from build123d import *

# Parameters (mm, degrees)
ESQUISSE1_R        = 10.75
BOSS_EXTRU_1_DEPTH = 6
ESQUISSE3_R        = 0.7
BOSS_EXTRU_2_DEPTH = 3
CONG_1_R           = 1


with BuildPart() as part:
    # Esquisse1 → Boss.-Extru.1 (new body)
    with BuildSketch(Plane.XY):
        Circle(ESQUISSE1_R)
    extrude(amount=BOSS_EXTRU_1_DEPTH)

    # Esquisse3 → Boss.-Extru.2 (add)
    with BuildSketch(Plane(origin=(0, 0, 0), x_dir=(-1, 0, 0), z_dir=(0, 0, -1))):
        with Locations(Location((-2.5, 0, 0), (0, 0, 180))):
            Circle(ESQUISSE3_R)
        with Locations(Location((2.5, 0, 0), (0, 0, 180))):
            Circle(ESQUISSE3_R)
    extrude(amount=BOSS_EXTRU_2_DEPTH)

    # Congé1
    cong_1_edges = [part.edges().sort_by_distance(p)[0] for p in [
        (-10.75, 0, 0),
        (-10.75, 0, 6),
    ]]
    fillet(cong_1_edges, radius=CONG_1_R)


solid = part.part
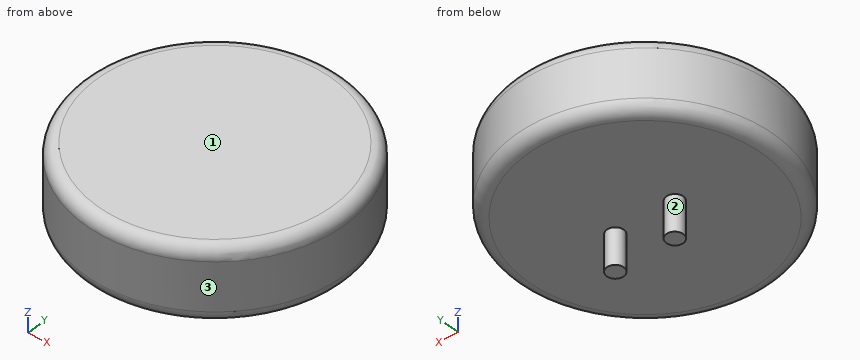
Can you work these out from the model? Positions are in its coordinate system, mm. Face numbers are marked on the shaded views. Round coordinates to 2 decimals unless told otherwise and drop trailing zeros. Write each loop counter-clockwise with the first axis right and the second up, starting at its lowest first coordinate (ties: lowest second). Pieces come first, ordered by that corner, then holes. Notation, with made-up numbers: (-24, 74.5) - (35, 74.5) arc R23 cw to (35, 92.5) - close; hole circle Ø4 at (-27, -8.75). An arc over 180 degrees is marked (long way). Write each question's results on one line, items separated by ' | '. Start each with the question number.
1) Please list where these lines run through material, in increasing order: line 1 (Z direction, x = 4.5, y = -4); line 2 (Y direction, x = -4.75, z = 0.5); line 3 (Y direction, x = 9.5, z = 1.5).
2) Suppose I cut it at C-C (z = -0.5). List the corners of the cut face in (x, y) for me, and give its area (3 significant figures).
3) Suppose I cut it at D-D (z = 2.25). List the corners of the cut face in (x, y) for me, and give its area (3 significant figures).
4) We'd pull the mould along X, two halves only. Please class the marked faces 1, 2 and 3: released by +X, released by -X, zero draft, split by the parting line, or undercut.
5) For pin 1 Ø2 at (x, z) = (3, 1) entering from -Y; pin 2 Ø1.5 at (x, z) = (1, 3) entering from -Y, each with a flat end and sliding along its axis, tell me the tip position at first contact or that it passes through.
6) Suppose I cut it at A-A (y = 0). List the corners of the cut face in (x, z) for me, and give its area (3 significant figures).
7) Suppose I cut it at B-B (x = 0). List the corners of the cut face in (y, z) for me.
Here are the results:
1) line 1: z = 0 to 6 | line 2: y = -9.49 to 9.49 | line 3: y = -5.03 to 5.03
2) outline: circle Ø1.4 at (-2.5, 0); circle Ø1.4 at (2.5, 0) | area: 3.08 mm2
3) outline: circle Ø21.5 at (0, 0) | area: 363 mm2
4) face 1: zero draft | face 2: undercut | face 3: split by the parting line
5) pin 1: stops at y = -10.56 | pin 2: stops at y = -10.75
6) outline: (-10.75, 1) arc R1 ccw to (-9.75, 0) - (-3.2, 0) - (-3.2, -3) - (-1.8, -3) - (-1.8, 0) - (1.8, 0) - (1.8, -3) - (3.2, -3) - (3.2, 0) - (9.75, 0) arc R1 ccw to (10.75, 1) - (10.75, 5) arc R1 ccw to (9.75, 6) - (-9.75, 6) arc R1 ccw to (-10.75, 5) - close | area: 137 mm2
7) outline: (-10.75, 1) arc R1 ccw to (-9.75, 0) - (9.75, 0) arc R1 ccw to (10.75, 1) - (10.75, 5) arc R1 ccw to (9.75, 6) - (-9.75, 6) arc R1 ccw to (-10.75, 5) - close
